Geometry check sheet. Reference: drawing and pictorial views, mm from the part's lowest x, y, z. A direction names the side the tool comes from. Round coordinates to 2 decimals unless told otherwise and drop trailing zeros. Write each loop counter-clockwise with the first axis right and the second up, starting at its lowest first coordinate (ties: lowest second). Pieces come first, ordered by that corner, then holes. Notation, with made-up numbers: (60, 79.5) - (100, 79.5) arc R24 cw to (100, 114.5) - close; hole circle Ø11 at (-16, 76). An arc over 180 degrees is marked (long way). Use one line per item in the form item = value. Start each with the question number.
1) Section check D-D (x = 51). Record the boundary of the cut face in (y, z).
2) Section check A-A (x = 40). Record the boundary of the cut face in (y, z).
3) Scan lines: probe 1 along Y at (x, z) = (44, 105); probe 2 along Z at (x, y) = (13, 12). Record each from-to range of solid material in increasing order.
4) Gauge pin test, flat ends, axial feed: P1, Ø2, axis at x = 54, z = 39, coming from the +Y side; P2, Ø6, axis at x = 8.5, y = 50.5, coming from the +Z side. Record the tip position at first contact, or that the pin passes through.
5) Section check B-B (z = 34). Record the boundary of the cut face in (x, y).
6) Set-up check for the marked faces 1 and 2: record each of +Z, -Z, +X, -X, +Y, -Y from which the full face is reachable in a straight line by a thin tool's end or side.
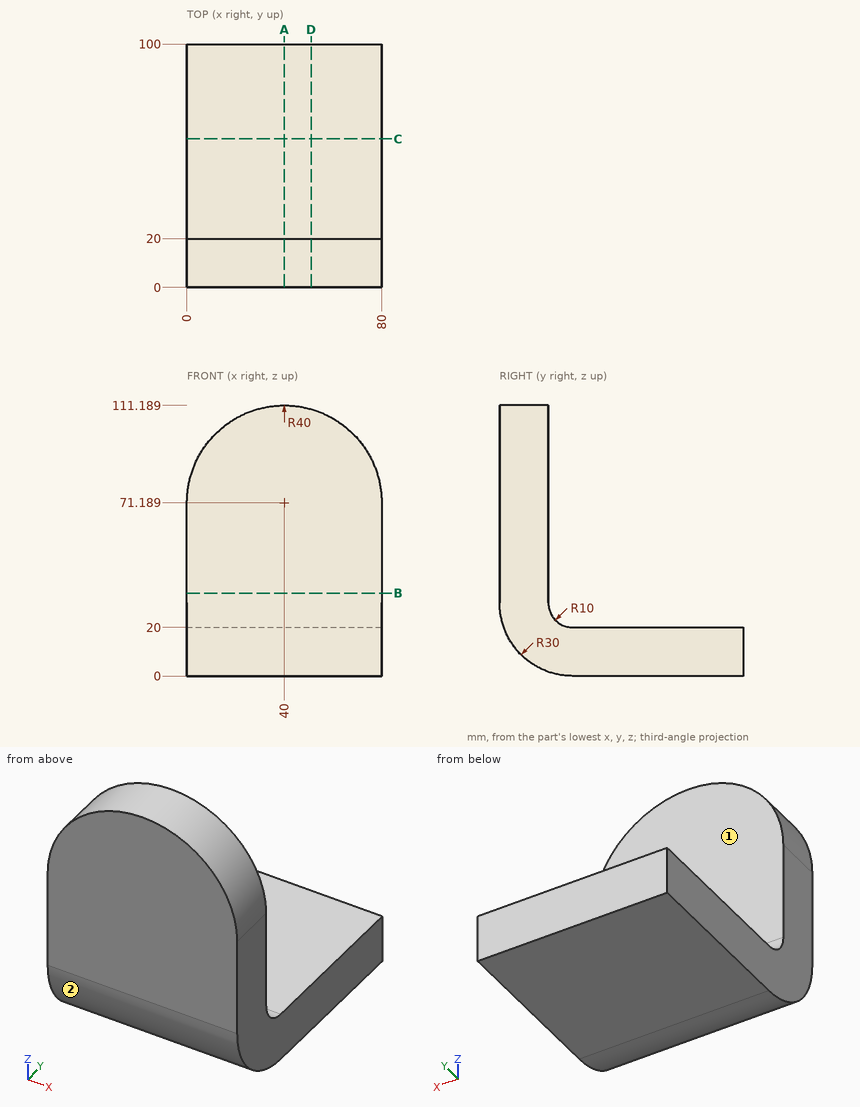
Results are:
q1.outline = (0, 30) arc R30 ccw to (30, 0) - (100, 0) - (100, 20) - (30, 20) arc R10 cw to (20, 30) - (20, 109.65) - (0, 109.65) - close
q2.outline = (0, 30) arc R30 ccw to (30, 0) - (100, 0) - (100, 20) - (30, 20) arc R10 cw to (20, 30) - (20, 111.19) - (0, 111.19) - close
q3.probe_1 = 0 to 20
q3.probe_2 = 6 to 100.7
q4.P1 = 20
q4.P2 = 20
q5.outline = (0, 0) - (80, 0) - (80, 20) - (0, 20) - close
q6.face_1 = +Z, +X, -X, +Y
q6.face_2 = -Z, +X, -X, -Y
